Check sheet for the modelled part. Datum: model origin and axes. Units: mm. Round coordinates to 2 decimals unless told otherwise and drop trailing zeros. Order: outer loops, then holes, each group sorted by start corner. A loop starts at its lowest first (then second) coordinate and runs counter-clockwise, first axis right, second up. Notation, with made-up numbers: (-9.5, 48.25) -> (15.5, 48.25) arc R9 ccw to (15.5, 52.25) -> close; hole circle Ø1 at (77, 56). An arc over 180 degrees is marked (long way). Answer in a Markdown table with one row per item.
```python
from build123d import *

# Parameters (mm, degrees)
BOSS_EXTRUDE1_DEPTH    = 12
F_12_0MM_DOWEL_HOLE1_D = 12


with BuildPart() as part:
    # Sketch1 → Boss-Extrude1 (new body)
    with BuildSketch(Plane(origin=(0, 0, 0), x_dir=(1, 0, 0), z_dir=(0, 1, 0))):
        Polygon((7.505553499, 13), (-7.505553499, 13), (-15.011106999, 0), (-7.505553499, -13), (7.505553499, -13), (15.011106999, 0), align=None)
    extrude(amount=BOSS_EXTRUDE1_DEPTH)

    # Ø12.0mm Dowel Hole1 (through all)
    with Locations(Plane(origin=(0, 0, 0), x_dir=(-1, 0, 0), z_dir=(0, -1, 0))):
        with Locations((0, 0)):
            Hole(F_12_0MM_DOWEL_HOLE1_D / 2)

    # Sketch4 → Cut-Revolve2 (revolve, cut)
    with BuildSketch(Plane.XY, mode=Mode.PRIVATE) as cut_revolve2_sk:
        with BuildLine():
            Line((19.381381373, -4.532480394), (19.381381373, 2.5))
            Line((19.381381373, 2.5), (15.011106999, 2.5))
            ThreePointArc((15.011106999, 2.5), (14.278873952, 0.732233047), (12.511106999, 0))
            Line((12.511106999, 0), (12.511106999, -4.532480394))
            Line((12.511106999, -4.532480394), (19.381381373, -4.532480394))
        make_face()
    cut_revolve2 = revolve(cut_revolve2_sk.sketch.rotate(Axis((0, 14.406395282, 0), (0, -1, 0)), 270), axis=Axis((0, 14.406395282, 0), (0, -1, 0)), mode=Mode.SUBTRACT)

    # Mirror1: Cut-Revolve2 across plane
    add(cut_revolve2.mirror(Plane(origin=(0, 6, 0), x_dir=(0, 0, 1), z_dir=(0, -1, 0))), mode=Mode.SUBTRACT)


solid = part.part
```
(1) Scan lines: probe 1 along Z at (x, y) = (0, 7); probe 2 along Z at (x, y) = (-4, 5); probe 3 along X at (y, z) = (8.25, -0.5). Record each from-to range of solid material in increasing order. Write a range as from..to.
Solutions:
| item | result |
|---|---|
| probe 1 | -13..-6, 6..13 |
| probe 2 | -13..-4.47, 4.47..13 |
| probe 3 | -14.72..-5.98, 5.98..14.72 |
(2) Section check B-B on y = 8.25. Record the boundary of the cut face in (x, z), plus the area to 3 significant figures.
Solutions:
| item | result |
|---|---|
| outline | (-15.01, 0) -> (-7.51, -13) -> (7.51, -13) -> (15.01, 0) -> (7.51, 13) -> (-7.51, 13) -> close; hole circle Ø12 at (0, 0) |
| area | 472 mm^2 |
(3) Draft check along Z on faces 1 (the flat face through (5.4, 0, -3)), 2 (the flat face through (11.2, 5.9, 6.6)), 3 (the flat face through (-11.2, 5.9, -6.6)), 4 (the cylindrical face through (-6, 6, 0)). Enter one of: pulls with the +Z half, pulls with the -Z half, needs draft (parallel to the pull), parting line crosses it, or undercut.
Solutions:
| item | result |
|---|---|
| face 1 | needs draft |
| face 2 | pulls with the +Z half |
| face 3 | pulls with the -Z half |
| face 4 | undercut |
(4) Depth check by flat-ended pin: pin 1 Ø1.5 at (y, z) = (8.5, 2.5) entering from +X. Enter the tip coordinate at first touch or a pass-through.
Solutions:
| item | result |
|---|---|
| pin 1 | x = 14 |
(5) Section check A-A on x = 0. Record the boundary of the cut face in (y, z), plus the area to 3 significant figures.
Solutions:
| item | result |
|---|---|
| outline | (0, -12.51) arc R2.5 ccw to (0.05, -13) -> (11.95, -13) arc R2.5 ccw to (12, -12.51) -> (12, -6) -> (0, -6) -> close; (0, 6) -> (12, 6) -> (12, 12.51) arc R2.5 ccw to (11.95, 13) -> (0.05, 13) arc R2.5 ccw to (0, 12.51) -> close |
| area | 168 mm^2 |
